```python
from build123d import *

# Parameters (mm, degrees)
F1_DEPTH     = 25.4
F2_T         = -2.54
F4_DEPTH     = 25.4
F5_T         = 2.54
F5_T3_DEPTH  = 30.48
F5_T5_DEPTH  = 10.9375095944
F5_T7_DEPTH  = 21.4331791904
F5_T9_DEPTH  = 11.5273250997
F5_T11_DEPTH = 11.5273250997
F5_T13_DEPTH = 11.5273250997
F5_T15_DEPTH = 11.5273250997
F5_T17_DEPTH = 11.5273250997
F5_T19_DEPTH = 11.5273250997
F5_T21_DEPTH = 11.5273250997
F5_T23_DEPTH = 11.5273250997
F5_T25_DEPTH = 11.5273250997
F5_T27_DEPTH = 11.5273250997
F5_T29_DEPTH = 11.5273250997
F5_T31_DEPTH = 5.7399744024
F5_T33_DEPTH = 17.6352883916
F5_T35_DEPTH = 25.6999516571
F5_T37_DEPTH = 25.6999516571
F5_T39_DEPTH = 5.8481406641
F5_T41_DEPTH = 30.48
F5_T43_DEPTH = 27.94


# Not quite as in the source:
# - a shell that OpenCascade refuses in one call is made with other operations: the cavity is built on its own and cut out


with BuildPart() as f1:
    # F0 (on Front) → F1 (new body)
    with BuildSketch(Plane.XZ):
        Polygon((76.6998529434, 0), (0, 75.1383975148), (-75.6014883518, 0), (-75.6014883518, -73.6595392227), (0, 0), align=None)
    extrude(amount=F1_DEPTH)

    # F2
    f2_openings = [f1.faces().sort_by_distance(p)[0] for p in [
        (-16.251734, -25.4, 8.81054),
    ]]
    offset(amount=F2_T, openings=f2_openings, kind=Kind.INTERSECTION)

    # F3 (on face) → F4 (join)
    with BuildSketch(Plane(origin=(0, 0, 0), x_dir=(-1, 0, 0), z_dir=(0, 1, 0))):
        Polygon((45.1430156827, -3.2236625498), (45.1430156827, 3.2236625498), (42.1467943112, 8.9324854087), (37.8800218445, 8.9324854087), (31.0955953813, 13.2925715491), (30.4404329353, 13.3721226726), (24.4120792452, 11.0858696839), (20.1367118865, 6.2599775498), (18.5937659974, 0), (20.1367118865, -6.2599775498), (24.4120792452, -11.0858696839), (30.4404329353, -13.3721226726), (36.8407497759, -12.5949835086), (42.1467943112, -8.9324854087), align=None)
        Polygon((37.8800218445, 8.9324854087), (42.1467943112, 8.9324854087), (36.8407497759, 12.5949835086), (31.0955953813, 13.2925715491), align=None)
        Polygon((36.8407497759, 12.5949835086), (42.1467943112, 8.9324854087), (58.4999735016, 8.9324854087), (75.8465806799, 20.0804729285), (84.4124181657, 38.8370406985), (81.4778930804, 59.2471109792), (67.9746964043, 74.8306306673), (48.189997673, 80.6399423696), (28.4052989418, 74.8306306673), (14.9021022657, 59.2471109792), (11.9675771804, 38.8370406985), (20.5334146661, 20.0804729285), (31.0955953813, 13.2925715491), align=None)
    extrude(amount=F4_DEPTH)

    # F5: shell of thickness 2.54, made by hand


with BuildPart() as f5_core1:
    # F5_t2: copy of F1
    add(f1.part)

    # the walls: a layer under each face that stays
    f5_faces = [f5_core1.faces().sort_by_distance(p)[0] for p in [
        (38.3499264717, -12.7, 37.5691987574),
        (38.3499264717, -12.7, 0),
        (-37.8007441759, -12.7, 37.5691987574),
        (0.5491822958, 0, 0.7394291461),
        (0.5491822958, -25.4, 0.7394291461),
        (-37.8007441759, -12.7, -36.8297696114),
        (-75.6014883518, -12.7, -36.8297696114),
        (-67.1732770908, 12.7, 14.5064791686),
        (-50.3233839064, 12.7, 8.9324854087),
        (-43.6449049969, 12.7, 6.0780739793),
        (-45.1430156827, 12.7, 0),
        (-43.6449049969, 12.7, -6.0780739793),
        (-39.4937720436, 12.7, -10.7637344586),
        (-33.6405913556, 12.7, -12.9835530906),
        (-27.4262560902, 12.7, -12.2289961783),
        (-22.2743955659, 12.7, -8.6729236169),
        (-19.365238942, 12.7, -3.1299887749),
        (-19.365238942, 12.7, 3.1299887749),
        (-22.2743955659, 12.7, 8.6729236169),
        (-27.4262560902, 12.7, 12.2289961783),
        (-30.7680141583, 12.7, 13.3323471109),
        (-25.8145050237, 12.7, 16.6865222388),
        (-16.2504959233, 12.7, 29.4587568135),
        (-13.434839723, 12.7, 49.0420758389),
        (-21.6537006037, 12.7, 67.0388708233),
        (35.245158445, -13.97, 37.0550334809),
        (34.7223268727, -13.97, 2.54),
        (-37.0471427298, -13.97, -32.5492576556),
        (-73.0614883518, -13.97, -34.3475958286),
        (-36.5243111575, -13.97, 35.2566953079),
        (-38.2976483074, 12.7, 77.7352865185),
        (-58.0823470387, 12.7, 77.7352865185),
        (-74.7262947424, 12.7, 67.0388708233),
        (-82.945155623, 12.7, 49.0420758389),
        (-80.1294994228, 12.7, 29.4587568135),
        (-48.189997673, 25.4, 33.6339098485),
    ]]
    thicken(f5_faces, amount=-F5_T, mode=Mode.SUBTRACT)

    # F5_s4 → F5_t3 (cut)
    with BuildSketch(Plane.XZ.offset(-2.54)):
        Polygon((0.0177253382, -0.0435926464), (0, 2.54), (-1.0327971077, 2.54), (-1.7725338247, 1.8192646427), align=None)
    extrude(amount=F5_T3_DEPTH, mode=Mode.SUBTRACT)

    # F5_s6 → F5_t5 (cut)
    with BuildSketch(Plane(origin=(-43.3267236667, 0, 27.8443945691), x_dir=(0, 1, 0), z_dir=(-0.8412535328, 0, 0.5406408175))):
        Polygon((0.0254, 24.138388588), (-2.54, 24.112988588), (-2.54, 21.572988588), (0, 21.572988588), align=None)
    extrude(amount=F5_T5_DEPTH, mode=Mode.SUBTRACT)

    # F5_s8 → F5_t7 (cut)
    with BuildSketch(Plane.YZ.offset(-61.0399735016)):
        Polygon((0.0254, 8.9070854087), (-2.54, 8.9324854087), (-2.54, 11.4724854087), (0, 11.4724854087), align=None)
    extrude(amount=F5_T7_DEPTH, mode=Mode.SUBTRACT)

    # F5_s10 → F5_t9 (cut)
    with BuildSketch(Plane(origin=(-9.6033156793, 0, -18.2975892876), x_dir=(0, 1, 0), z_dir=(0.464723172, 0, 0.8854560257))):
        Polygon((0.0254, 41.4956659382), (-2.54, 41.4702659382), (-2.54, 38.9302659382), (0, 38.9302659382), align=None)
    extrude(amount=F5_T9_DEPTH, mode=Mode.SUBTRACT)

    # F5_s12 → F5_t11 (cut)
    with BuildSketch(Plane.XY.offset(-5.7636625498)):
        Polygon((-45.1684156827, 0.0254), (-45.1430156827, -2.54), (-42.6030156827, -2.54), (-42.6030156827, 0), align=None)
    extrude(amount=F5_T11_DEPTH, mode=Mode.SUBTRACT)

    # F5_s14 → F5_t13 (cut)
    with BuildSketch(Plane(origin=(-4.2463005938, 0, 8.0906498184), x_dir=(0, 1, 0), z_dir=(-0.464723172, 0, 0.8854560257))):
        Polygon((0.0254, 41.4956659382), (-2.54, 41.4702659382), (-2.54, 38.9302659382), (0, 38.9302659382), align=None)
    extrude(amount=F5_T13_DEPTH, mode=Mode.SUBTRACT)

    # F5_s16 → F5_t15 (cut)
    with BuildSketch(Plane(origin=(-16.9736937466, 0, 11.7160948578), x_dir=(0, 1, 0), z_dir=(-0.8229838659, 0, 0.5680647467))):
        Polygon((0.0254, 31.3187994096), (-2.54, 31.2933994096), (-2.54, 28.7533994096), (0, 28.7533994096), align=None)
    extrude(amount=F5_T15_DEPTH, mode=Mode.SUBTRACT)

    # F5_s18 → F5_t17 (cut)
    with BuildSketch(Plane(origin=(-25.876601356, 0, 3.1419882557), x_dir=(0, 1, 0), z_dir=(-0.9927088741, 0, 0.1205366803))):
        Polygon((0.0254, 16.9692135742), (-2.54, 16.9438135742), (-2.54, 14.4038135742), (0, 14.4038135742), align=None)
    extrude(amount=F5_T17_DEPTH, mode=Mode.SUBTRACT)

    # F5_s20 → F5_t19 (cut)
    with BuildSketch(Plane(origin=(-22.6430959031, 0, -8.5873935644), x_dir=(0, 1, 0), z_dir=(-0.9350162427, 0, -0.354604887))):
        Polygon((0.0254, 1.7342256155), (-2.54, 1.7088256155), (-2.54, -0.8311743845), (0, -0.8311743845), align=None)
    extrude(amount=F5_T19_DEPTH, mode=Mode.SUBTRACT)

    # F5_s22 → F5_t21 (cut)
    with BuildSketch(Plane(origin=(-10.277585823, 0, -11.6009962232), x_dir=(0, 1, 0), z_dir=(-0.6631226582, 0, -0.7485107482))):
        Polygon((0.0254, -10.8960123265), (-2.54, -10.9214123265), (-2.54, -13.4614123265), (0, -13.4614123265), align=None)
    extrude(amount=F5_T21_DEPTH, mode=Mode.SUBTRACT)

    # F5_s24 → F5_t23 (cut)
    with BuildSketch(Plane(origin=(-0.4570401404, 0, -1.854284741), x_dir=(0, 1, 0), z_dir=(-0.2393156643, 0, -0.9709418174))):
        Polygon((0.0254, -18.0280649503), (-2.54, -18.0534649503), (-2.54, -20.5934649503), (0, -20.5934649503), align=None)
    extrude(amount=F5_T23_DEPTH, mode=Mode.SUBTRACT)

    # F5_s26 → F5_t25 (cut)
    with BuildSketch(Plane(origin=(-3.2157096041, 0, 13.0466467234), x_dir=(0, 1, 0), z_dir=(0.2393156643, 0, -0.9709418174))):
        Polygon((0.0254, -18.0280649503), (-2.54, -18.0534649503), (-2.54, -20.5934649503), (0, -20.5934649503), align=None)
    extrude(amount=F5_T25_DEPTH, mode=Mode.SUBTRACT)

    # F5_s28 → F5_t27 (cut)
    with BuildSketch(Plane(origin=(-17.9216162855, 0, 20.229322958), x_dir=(0, 1, 0), z_dir=(0.6631226582, 0, -0.7485107482))):
        Polygon((0.0254, -10.8960123265), (-2.54, -10.9214123265), (-2.54, -13.4614123265), (0, -13.4614123265), align=None)
    extrude(amount=F5_T27_DEPTH, mode=Mode.SUBTRACT)

    # F5_s30 → F5_t29 (cut)
    with BuildSketch(Plane(origin=(-33.4213321061, 0, 12.6750393793), x_dir=(0, 1, 0), z_dir=(0.9350162427, 0, -0.354604887))):
        Polygon((0.0254, 1.7342256155), (-2.54, 1.7088256155), (-2.54, -0.8311743845), (0, -0.8311743845), align=None)
    extrude(amount=F5_T29_DEPTH, mode=Mode.SUBTRACT)

    # F5_s32 → F5_t31 (cut)
    with BuildSketch(Plane(origin=(-31.5747248824, 0, -3.8338657149), x_dir=(0, 1, 0), z_dir=(0.9927088741, 0, 0.1205366803))):
        Polygon((0.0254, 16.9692135742), (-2.54, 16.9438135742), (-2.54, 14.4038135742), (0, 14.4038135742), align=None)
    extrude(amount=F5_T31_DEPTH, mode=Mode.SUBTRACT)

    # F5_s34 → F5_t33 (cut)
    with BuildSketch(Plane(origin=(-3.2619473911, 0, -2.0963262978), x_dir=(0, 1, 0), z_dir=(-0.8412535328, 0, -0.5406408175))):
        Polygon((0.0254, -27.9685708823), (-2.54, -27.9939708823), (-2.54, -30.5339708823), (0, -30.5339708823), align=None)
    extrude(amount=F5_T33_DEPTH, mode=Mode.SUBTRACT)

    # F5_s36 → F5_t35 (cut)
    with BuildSketch(Plane(origin=(13.6654522193, 0, 29.9231664254), x_dir=(0, 1, 0), z_dir=(-0.415415013, 0, -0.9096319954))):
        Polygon((0.0254, -26.9941808769), (-2.54, -27.0195808769), (-2.54, -29.5595808769), (0, -29.5595808769), align=None)
    extrude(amount=F5_T35_DEPTH, mode=Mode.SUBTRACT)

    # F5_s38 → F5_t37 (cut)
    with BuildSketch(Plane(origin=(-9.0092196449, 0, 62.6604989846), x_dir=(0, 1, 0), z_dir=(0.1423148383, 0, -0.9898214419))):
        Polygon((0.0254, -6.2932773345), (-2.54, -6.3186773345), (-2.54, -8.8586773345), (0, -8.8586773345), align=None)
    extrude(amount=F5_T37_DEPTH, mode=Mode.SUBTRACT)

    # F5_s40 → F5_t39 (cut)
    with BuildSketch(Plane(origin=(-37.8790578276, 0, 43.7147630729), x_dir=(0, 1, 0), z_dir=(0.6548607339, 0, -0.7557495744))):
        Polygon((0.0254, 27.5617491357), (-2.54, 27.5363491357), (-2.54, 24.9963491357), (0, 24.9963491357), align=None)
    extrude(amount=F5_T39_DEPTH, mode=Mode.SUBTRACT)

    # F5_s42 → F5_t41 (cut)
    with BuildSketch(Plane.XZ.offset(-27.94)):
        Polygon((-42.1692848942, 8.9188893773), (-42.1467943112, 11.4724854087), (-37.9451211064, 11.4724854087), (-39.897736006, 7.7520885517), align=None)
        Polygon((-31.0849247362, 13.2964185148), (-30.7894322134, 10.7710910089), (-41.7969422831, 9.4345373059), (-32.4688230576, 15.4293555225), align=None)
    extrude(amount=F5_T41_DEPTH, mode=Mode.SUBTRACT)

    # F5_s44 → F5_t43 (cut)
    with BuildSketch(Plane.XZ):
        Polygon((70.4596759808, 2.5472557471), (72.254938082, 4.3544252949), (76.6998529434, 0), (70.4774508531, 0), align=None)
        Polygon((0.0129964155, 71.5339071047), (1.7903532658, 73.3844922566), (0, 75.1383975148), (-1.7776590552, 73.3716273672), align=None)
        Polygon((-73.0538136901, -67.6203226649), (-71.2889545271, -69.457779954), (-75.6014883518, -73.6595392227), (-75.6014883518, -67.6385153113), align=None)
        Polygon((-73.0181831009, -1.0746919499), (-75.6014883518, -1.0566763458), (-75.6014883518, 0), (-74.8520134439, 0.7448840596), align=None)
    extrude(amount=F5_T43_DEPTH, mode=Mode.SUBTRACT)


with BuildPart() as f1_1:
    add(f1.part)

    # what is left inside the walls is the cavity
    f5_cavity = [f5_core1.part.solids().sort_by_distance(p)[0] for p in [
        (-48.189998, 22.8346, 33.645894),
        (-31.906399, 22.8346, -3.591727),
    ]]
    add(f5_cavity, mode=Mode.SUBTRACT)


solid = f1_1.part
```
Geometry check sheet. Reference: the model listing, model coordinates, mm. A direction names the side the tool comes from. Give positions to 0.01 mm unless a question says otherwise; leave off trailing zeros. Write each loop counter-clockwise with the first axis right and the second up, starting at its lowest first coordinate (ties: lowest second). Pieces come first, ordered by that corner, then holes. Notation, with made-up numbers: (61, 72) -> (120, 72) arc R19 cw to (120, 108) -> close; hole circle Ø10 at (1, -13.5). An arc over 180 degrees is marked (long way). One line per question, with ' | ' between items.
Item 1: Depth check by flat-ended pin: pin 1 (6.5 mm diameter, centred on x = -36.5, z = 3, fed in from -Y); pin 2 (1.5 mm diameter, centred on x = 57.5, z = 16.5, fed in from +Y); pin 3 (1.5 mm diameter, centred on y = -12, z = 47, fed in from -X). Enter the tip coordinate at first touch or a pass-through.
Determined:
pin 1: y = 22.86 | pin 2: y = 0 | pin 3: x = -29.07
Item 2: Scan lines: line 1 along Z through (x, y) = (-43, 5.5); line 2 along Z through (x, y) = (-44, 6.5); line 3 along Y through (x, z) = (-65.5, -34.5). Record each from-to range of solid material in increasing order.
Determined:
line 1: -7.31 to 7.31, 8.93 to 11.47, 76.47 to 79.12 | line 2: -5.4 to 5.4, 8.93 to 11.47, 76.76 to 79.41 | line 3: -2.54 to 0
Item 3: Sectioned sample at A-A, the plane y = -17. Record the boundary of the cut face in (x, z).
Determined:
outline: (-75.6, -73.66) -> (0, 0) -> (76.7, 0) -> (0, 75.14) -> (-75.6, 0) -> close; hole (-73.06, -67.64) -> (-1.03, 2.54) -> (70.48, 2.54) -> (0.01, 71.57) -> (-73.06, -1.06) -> close
Item 4: Sectioned sample at D-D, the plane y = 7. State how many separate pieces and enclosed holes the cut face has, plus the area to 3 significant figures.
Determined:
separate pieces: 1 | enclosed holes: 2 | area: 726 mm^2
Item 5: Sectioned sample at B-B, the plane z = -31.5. Record the boundary of the cut face in (x, y).
Determined:
outline: (-75.6, -25.4) -> (-73.06, -25.4) -> (-73.06, -2.54) -> (-35.97, -2.54) -> (-35.97, -25.4) -> (-32.33, -25.4) -> (-32.33, 0) -> (-75.6, 0) -> close
Item 6: Draft check along X on faces 1 (the flat face through (-32, 22.86, 0)), 2 (the flat face through (-80.07, 12.52, 29.33)), 3 (the flat face through (-22.244, 12.522, -8.639)). Enter one of: released by +X, released by -X, zero draft, split by the parting line, or undercut.
Determined:
face 1: undercut | face 2: released by -X | face 3: released by +X
Item 7: Access from +Z, -Z, +X, -X, +Y, -Y to the whole of each face (thin tool, end or side, straight path). Record for faces 4 (the flat face through (-33.6, 12.52, -12.99)), 5 (the flat face through (-27.468, 12.522, 12.245)), 6 (the flat face through (34, -14, 2.54)).
Determined:
face 4: -Z, -X, +Y | face 5: +X, +Y | face 6: -Y
Item 8: Sectioned sample at C-C, the plane x = 66.5. Record the boundary of the cut face in (y, z).
Determined:
outline: (-25.4, 0) -> (0, 0) -> (0, 9.99) -> (-25.4, 9.99) -> (-25.4, 6.44) -> (-2.54, 6.44) -> (-2.54, 2.54) -> (-25.4, 2.54) -> close
